Can you work these out from the model? Positions are in its coordinate system, mm. A direction names the side the tool comes from. Round coordinates to 2 decimals unless told otherwise and drop trailing zeros. Order: outer loops, then holes, each group sorted by start corner. A loop starts at its lowest first (then second) coordinate and runs counter-clockwise, first axis right, second up. Notation, with made-up numbers: (-25.5, 38) -> (26.5, 38) arc R19 ccw to (26.5, 74) -> close; hole circle Ø11 at (-29, 23.25). An arc over 180 degrees is marked (long way). One line per item, written item: value.
```python
from build123d import *

# Parameters (mm, degrees)
BOSS_EXTRUDE1_DEPTH = 15
SKETCH5_W           = 155.5
SKETCH5_H           = 155.5
CUT_EXTRUDE3_DEPTH  = 11
SKETCH7_R           = 1.75
CUT_EXTRUDE4_DEPTH  = 2.5


with BuildPart() as part:
    # Sketch1 → Boss-Extrude1 (new body)
    with BuildSketch(Plane(origin=(0, 0, 0), x_dir=(1, 0, 0), z_dir=(0, 1, 0))):
        Polygon((20, 159.5), (0, 139.5), (0, 20), (20, 0), (139.5, 0), (159.5, 20), (159.5, 139.5), (139.5, 159.5), align=None)
    extrude(amount=BOSS_EXTRUDE1_DEPTH)

    # Sketch5 → Cut-Extrude3 (cut)
    with BuildSketch(Plane.XZ):
        with Locations((79.75, -79.75)):
            Rectangle(SKETCH5_W, SKETCH5_H)
    extrude(amount=-CUT_EXTRUDE3_DEPTH, mode=Mode.SUBTRACT)

    # Sketch7 → Cut-Extrude4 (cut)
    with BuildSketch(Plane(origin=(0, 15, 0), x_dir=(1, 0, 0), z_dir=(0, 1, 0))):
        with Locations(Location((54.75, 114.75, 0), (0, 0, 270))):
            Circle(SKETCH7_R)
        with Locations(Location((104.75, 114.75, 0), (0, 0, 90))):
            Circle(SKETCH7_R)
        with Locations(Location((69.75, 114.75, 0), (0, 0, 270))):
            Circle(SKETCH7_R)
        with Locations(Location((88.92664449, 114.75, 0), (0, 0, 270))):
            Circle(SKETCH7_R)
        with Locations(Location((54.75, 84.75, 0), (0, 0, 270))):
            Circle(SKETCH7_R)
        with Locations(Location((69.75, 84.75, 0), (0, 0, 270))):
            Circle(SKETCH7_R)
        with Locations(Location((88.92664449, 84.75, 0), (0, 0, 270))):
            Circle(SKETCH7_R)
        with Locations(Location((104.75, 84.75, 0), (0, 0, 90))):
            Circle(SKETCH7_R)
    extrude(amount=-CUT_EXTRUDE4_DEPTH, mode=Mode.SUBTRACT)


solid = part.part
```
Q1. I want a section at C-C on z = -111. List the corners of the cut face in (x, y) for me.
Answers below:
outline: (0, 0) -> (2, 0) -> (2, 11) -> (157.5, 11) -> (157.5, 0) -> (159.5, 0) -> (159.5, 15) -> (0, 15) -> close
Q2. I want a section at B-B on x = 61. List the corners of the cut face in (y, z) for me, plus the area to 3 significant figures.
Answers below:
outline: (0, -159.5) -> (15, -159.5) -> (15, 0) -> (0, 0) -> (0, -2) -> (11, -2) -> (11, -157.5) -> (0, -157.5) -> close
area: 682 mm^2
Q3. On a 3-axis mill with a long thin cutter (end or side, diameter ignored), from which of +Z, -Z, +X, -X, +Y, -Y can I reach the whole of each face in a straight line? I mean faces 4 (the face through (157.5, 5, -81)), 5 (the face through (89, 12.5, -115)), 6 (the face through (79, 5, -157.5)), 7 (the face through (79, 11, -79)). Say none if no direction works.
Answers below:
face 4: +Z, -Z, -Y
face 5: +Y
face 6: +X, -X, -Y
face 7: -Y
Q4. I want a section at D-D on x = 150. List the corners of the cut face in (y, z) for me, plus the area to 3 significant figures.
Answers below:
outline: (11, -149) -> (15, -149) -> (15, -10.5) -> (11, -10.5) -> close
area: 554 mm^2
Q5. We'd pull the mould along Z, two halves only. Please class faces 1 (the face through (79, 15, -81)), 2 (the face through (79, 7, 0)), 3 (the face through (105, 12.5, -115)): released by +Z, released by -Z, zero draft, split by the parting line, or undercut.
Answers below:
face 1: zero draft
face 2: released by +Z
face 3: undercut
Q6. I want a section at A-A on y = 2.5. List the corners of the cut face in (x, z) for me.
Answers below:
outline: (0, -139.5) -> (2, -141.5) -> (2, -18) -> (0, -20) -> close; (18, -157.5) -> (20, -159.5) -> (139.5, -159.5) -> (141.5, -157.5) -> close; (18, -2) -> (141.5, -2) -> (139.5, 0) -> (20, 0) -> close; (157.5, -141.5) -> (159.5, -139.5) -> (159.5, -20) -> (157.5, -18) -> close
Q7. Will these pins go through, and if not, where does the flat tip stop? pin 1 Ø1.8 at (x, z) = (69.5, -84) entering from +Y; pin 2 Ø3 at (x, z) = (69.75, -84.75) entering from -Y; pin 3 Ø5 at (x, y) = (17, 12) entering from -Z.
Answers below:
pin 1: y = 12.5
pin 2: y = 11
pin 3: z = -159
Q8. Please list where these lines run through material, in increasing order: line 1 along X through (y, z) = (4, -137); line 2 along X through (y, z) = (13.45, -84.75); line 3 along Z through (x, y) = (68.5, 2.5).
Answers below:
line 1: 0 to 2, 157.5 to 159.5
line 2: 0 to 53, 56.5 to 68, 71.5 to 87.18, 90.68 to 103, 106.5 to 159.5
line 3: -159.5 to -157.5, -2 to 0
